```python
from build123d import *

# Parameters (mm, degrees)
F0_R     = 15.708112
F1_DEPTH = 25.4


with BuildPart() as f1:
    # F0 (on Top) → F1 (new body)
    with BuildSketch(Plane.XY):
        with BuildLine():
            ThreePointArc((8.357053, 27.856014), (10.344975, 31.219382), (11.036502, 35.064623))
            ThreePointArc((11.036502, 35.064623), (-0.452947, 46.091827), (-10.999324, 34.159493))
            ThreePointArc((-10.999324, 34.159493), (-3.417435, 24.570552), (8.357053, 27.856014))
        make_face()
        with BuildLine():
            ThreePointArc((8.357053, 27.856014), (-3.417435, 24.570552), (-10.999324, 34.159493))
            ThreePointArc((-10.999324, 34.159493), (-15.69672, 12.059533), (-28.302542, -6.690586))
            ThreePointArc((-28.302542, -6.690586), (-21.864291, -10.49592), (-19.330352, -17.532311))
            ThreePointArc((-19.330352, -17.532311), (-20.590542, -22.65365), (-24.083327, -26.60544))
            ThreePointArc((-24.083327, -26.60544), (-2.595502, -19.623525), (19.945489, -21.165427))
            ThreePointArc((19.945489, -21.165427), (22.987439, -9.325691), (35.082651, -7.554053))
            ThreePointArc((35.082651, -7.554053), (18.292222, 7.563992), (8.357053, 27.856014))
        make_face()
        Circle(F0_R, mode=Mode.SUBTRACT)
        with BuildLine():
            ThreePointArc((-19.330352, -17.532311), (-21.864291, -10.49592), (-28.302542, -6.690586))
            ThreePointArc((-28.302542, -6.690586), (-41.163704, -19.819761), (-24.083327, -26.60544))
            ThreePointArc((-24.083327, -26.60544), (-20.590542, -22.65365), (-19.330352, -17.532311))
        make_face()
        with BuildLine():
            ThreePointArc((41.403357, -17.532311), (39.69022, -11.626446), (35.082651, -7.554053))
            ThreePointArc((35.082651, -7.554053), (22.987439, -9.325691), (19.945489, -21.165427))
            ThreePointArc((19.945489, -21.165427), (32.209266, -28.413943), (41.403357, -17.532311))
        make_face()
    extrude(amount=F1_DEPTH)


solid = f1.part
```
Verification items for the finished model (mm, model axes). Coordinates: 2 decimals unless noted, no trailing zeros. Write each loop counter-clockwise with the first axis right and the second up, starting at its lowest first coordinate (ties: lowest second). Pieces come first, ordered by that corner, then holes. Notation, with made-up numbers: M 40,-0.5 L 73,-0.5 A15 cw 73,5.5 Z; hole C 64,42 d10. An arc over 180 degrees is marked long. Answer as a JSON object with one key per item and string values. Group by question number.
(1) Cross-section at D-D, the plane z = 10.25. Record the cut outline in (x, y).
(2) Gauge pin test, flat ends, axial feed: pin 1 (25 mm diameter, centred on x = 0, y = 0, fed in from +Z); pin 2 (2 mm diameter, centred on y = 28.5, z = 6.5, fed in from +X); pin 3 (1 mm diameter, centred on x = 29, z = 22, fed in from -Y); pin 4 (4 mm diameter, centred on y = 14, z = 7.5, fed in from -X). Record the tip position at first contact, or that the pin passes through.
(3) Cross-section at A-A, the plane y = -12. Record the cut outline in (x, z), and give its area (3 significant figures).
(4) Cross-section at B-B, the plane x = 9.5. Record the cut outline in (y, z), and give its area (3 significant figures).
(5) Cross-section at C-C, the plane x = 0. Record the cut outline in (y, z), and give its area (3 significant figures).
(6) Material ranges on line 1 (Y direction, x = 0, z = 7); line 2 (X direction, y = 4, z = 18.5); line 3 (X direction, y = 6, z = 10.25), recorded low to high.
(7) Release check for a two-part mould opening along X. For faces 1 (the face through (18.485, 7.31, 12.522)), 2 (the face through (-9.4, -13.2, 0)), 3 (the face through (-2.911, -19.663, 12.522)), 4 (the face through (-12.465, -9.558, 12.522)) record: +X half, -X half, draft (parallel to the pull), parting line (faces both ways), or undercut.
Reply:
{
 "1": {"outline": "M -28.3,-6.69 A11.04 ccw long -24.08,-26.61 A59.44 cw 19.95,-21.17 A11.04 ccw 41.4,-17.53 A11.04 ccw 35.08,-7.55 A59.44 cw 8.36,27.86 A11.04 ccw 11.04,35.06 A11.04 ccw long -11,34.16 A59.44 cw Z; hole C 0,0 d31.42"},
 "2": {"pin 1": "through", "pin 2": "x = 9.53", "pin 3": "y = -28.53", "pin 4": "x = -15.72"},
 "3": {"outline": "M -39.92,0 L -10.14,0 L -10.14,25.4 L -39.92,25.4 Z; M 10.14,0 L 39.92,0 L 39.92,25.4 L 10.14,25.4 Z", "area": "1,510 mm²"},
 "4": {"outline": "M -19.37,0 L -12.51,0 L -12.51,25.4 L -19.37,25.4 Z; M 12.51,0 L 24.12,0 L 24.12,25.4 L 12.51,25.4 Z; M 29.45,0 L 40.68,0 L 40.68,25.4 L 29.45,25.4 Z", "area": "755 mm²"},
 "5": {"outline": "M -19.36,0 L -15.71,0 L -15.71,25.4 L -19.36,25.4 Z; M 15.71,0 L 46.1,0 L 46.1,25.4 L 15.71,25.4 Z", "area": "865 mm²"},
 "6": {"line 1": "-19.36 to -15.71, 15.71 to 46.1", "line 2": "-19.86 to -15.19, 15.19 to 21.21", "line 3": "-18.68 to -14.52, 14.52 to 19.51"},
 "7": {"face 1": "+X half", "face 2": "draft", "face 3": "undercut", "face 4": "undercut"}
}
